Verification items for the finished model (mm, model axes). Face numbers are marked on the shaded views. A direction names the side the tool comes from. Round coordinates to 2 decimals unless told otherwise and drop trailing zeros. Order: outer loops, then holes, each group sorted by start corner. A loop starts at its lowest first (then second) coordinate and runs counter-clockwise, first axis right, second up. Notation, with made-up numbers: (-17, 51.25) -> (28, 51.25) arc R22 cw to (28, 86.25) -> close; hole circle Ø4 at (62, 83.5). An arc over 180 degrees is marked (long way). Put each result on its own line as item: value.
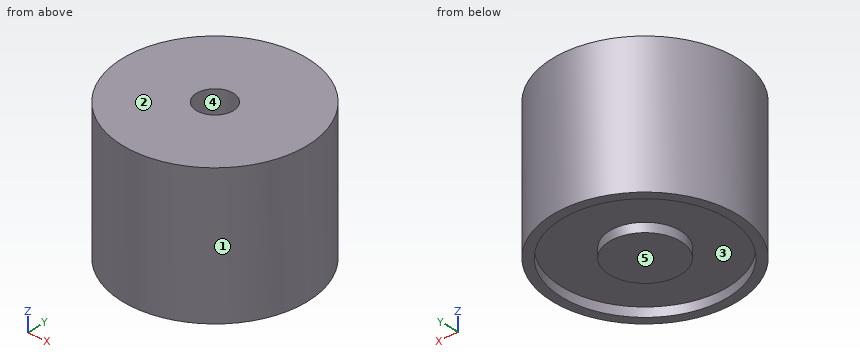
from build123d import *

# Parameters (mm, degrees)
CYLINDER033_R                = 2
CYLINDER033_DEPTH            = 5
TUBE_R                       = 9
TUBE_R_2                     = 3.85
TUBE_DEPTH                   = 1
CYLINDER032_R                = 10
CYLINDER032_DEPTH            = 15
CUT002002004_PLACEMENT_ANGLE = 180


with BuildPart() as cylinder033:
    # Cylinder033 → Cylinder033 (new body)
    with BuildSketch(Plane.XY):
        Circle(CYLINDER033_R)
    extrude(amount=CYLINDER033_DEPTH)


with BuildPart() as fusion014:
    # Tube → Tube (new body)
    with BuildSketch(Plane.XY.offset(14)):
        Circle(TUBE_R)
        Circle(TUBE_R_2, mode=Mode.SUBTRACT)
    extrude(amount=TUBE_DEPTH)

    # Fusion014: union Cylinder033
    add(cylinder033.part)


with BuildPart() as electromagnet:
    # Cylinder032 → Cylinder032 (new body)
    with BuildSketch(Plane.XY):
        Circle(CYLINDER032_R)
    extrude(amount=CYLINDER032_DEPTH)

    # Cut002002004: cut Fusion014
    add(fusion014.part, mode=Mode.SUBTRACT)


with BuildPart() as electromagnet_1:
    # Cut002002004 placement: moved
    add(electromagnet.part.moved(Location((-60, 15, -15))).rotate(Axis((-60, 15, -15), (1, 0, 0)), CUT002002004_PLACEMENT_ANGLE))


solid = electromagnet_1.part
Item 1: Gauge pin test, flat ends, axial feed: pin 1 Ø1.5 at (y, z) = (10, -26) entering from +X; pin 2 Ø8 at (x, z) = (-65, -21) entering from +Y; pin 3 Ø2 at (x, z) = (-67, -23.5) entering from -Y. Record the tip position at first contact, or that the pin passes through.
Check sheet entries:
pin 1: stops at x = -50.95
pin 2: stops at y = 24.95
pin 3: stops at y = 7
Item 2: Section check C-C on z = -16.25. Record the boundary of the cut face in (x, y), then the cut area to 3 significant figures.
Check sheet entries:
outline: circle Ø20 at (-60, 15); hole circle Ø4 at (-60, 15)
area: 302 mm^2
Item 3: Section check B-B on y = 15. Record the boundary of the cut face in (x, z).
Check sheet entries:
outline: (-70, -30) -> (-69, -30) -> (-69, -29) -> (-63.85, -29) -> (-63.85, -30) -> (-56.15, -30) -> (-56.15, -29) -> (-51, -29) -> (-51, -30) -> (-50, -30) -> (-50, -15) -> (-58, -15) -> (-58, -20) -> (-62, -20) -> (-62, -15) -> (-70, -15) -> close
Item 4: Section check A-A on x = -60. Record the boundary of the cut face in (y, z).
Check sheet entries:
outline: (5, -30) -> (6, -30) -> (6, -29) -> (11.15, -29) -> (11.15, -30) -> (18.85, -30) -> (18.85, -29) -> (24, -29) -> (24, -30) -> (25, -30) -> (25, -15) -> (17, -15) -> (17, -20) -> (13, -20) -> (13, -15) -> (5, -15) -> close
Item 5: Release check for a two-part mould opening along Y. For the marked faces 1, 2 and 3 record: +Y half, -Y half, draft (parallel to the pull), parting line (faces both ways), or undercut.
Check sheet entries:
face 1: parting line
face 2: draft
face 3: undercut
Item 6: Material ranges on L1, parallel to X at y = 15, z = -29.7; L2, parallel to Y at x = -60, z = -29.15; L3, parallel to Y at x = -60, z = -18.9, recorded low to high. Write a range as [from, to].
Check sheet entries:
L1: x = [-70, -69], [-63.85, -56.15], [-51, -50]
L2: y = [5, 6], [11.15, 18.85], [24, 25]
L3: y = [5, 13], [17, 25]
Item 7: Tool access check on the marked faces 4 and 5. Record the directions out of +Z, -Z, +X, -X, +Y, -Y that give a thin tool (end or side, any length) a straight path to the whole face; none if there is none.
Check sheet entries:
face 4: +Z
face 5: -Z, +X, -X, +Y, -Y
Item 8: Section check D-D on x = -62.75. Record the boundary of the cut face in (y, z).
Check sheet entries:
outline: (5.39, -30) -> (6.43, -30) -> (6.43, -29) -> (12.31, -29) -> (12.31, -30) -> (17.69, -30) -> (17.69, -29) -> (23.57, -29) -> (23.57, -30) -> (24.61, -30) -> (24.61, -15) -> (5.39, -15) -> close
